```python
from build123d import *

# Parameters (mm, degrees)
SKETCH1_W           = 1.5875
SKETCH1_H           = 177.8
BOSS_EXTRUDE1_DEPTH = 304.8
CUT_EXTRUDE1_DEPTH  = 1.5875
FILLET1_R           = 6.35


with BuildPart() as part:
    # Sketch1 → Boss-Extrude1 (new body)
    with BuildSketch(Plane(origin=(0, 0, 0), x_dir=(1, 0, 0), z_dir=(0, 1, 0))):
        with Locations((0.79375, 88.9)):
            Rectangle(SKETCH1_W, SKETCH1_H)
    extrude(amount=BOSS_EXTRUDE1_DEPTH)

    # Sketch2 → Cut-Extrude1 (cut)
    with BuildSketch(Plane.ZY):
        Polygon((-177.8, 25.4), (0, 304.8), (-177.8, 304.8), align=None)
    extrude(amount=-CUT_EXTRUDE1_DEPTH, mode=Mode.SUBTRACT)

    # Fillet1
    fillet1_edges = [part.edges().sort_by_distance(p)[0] for p in [
        (0.79375, 25.4, -177.8),
        (0.79375, 304.8, 0),
        (0.79375, 0, -177.8),
        (0.79375, 0, 0),
    ]]
    fillet(fillet1_edges, radius=FILLET1_R)


solid = part.part
```
Geometry: final body of the model. Coordinates: model frame, mm. Coordinates: 2 decimals unless noted, no trailing zeros. Loops run counter-clockwise (first coordinate to the right, second up) from the corner with the lowest first, then second, coordinate; pieces in that order, holes last. Notation, with made-up numbers: (75, -19) -> (111, -19) arc R10 cw to (111, -5) -> close; hole circle Ø9 at (25.25, -17.75). An arc over 180 degrees is marked (long way). Use a Markdown table: item, result. Add a question column.
(1) Line query: line 1 along Y through (x, z) = (1.4, -74); line 2 along Y through (x, z) = (0.75, -12); line 3 along Z through (x, y) = (0.7, 122). Output: solid intervals per line, ascending.
(2) Section query A-A, the plane x = 1.3. Return loops of the section in (y, z), plus the area to 3 significant figures.
(3) Section query C-C, the plane y = 248.5. Return loops of the section in (x, z).
(4) Section query B-B, the plane z = -66.5. Return loops of the section in (x, y), plus the area to 3 significant figures.
Answer:
| question | item | result |
|---|---|---|
| 1 | line 1 | y = 0 to 188.51 |
| 1 | line 2 | y = 0 to 285.94 |
| 1 | line 3 | z = -116.33 to 0 |
| 2 | outline | (0, -171.45) arc R6.35 ccw to (6.35, -177.8) -> (23.55, -177.8) arc R6.35 ccw to (26.96, -176.81) -> (286.4, -11.71) arc R6.35 ccw to (282.99, 0) -> (6.35, 0) arc R6.35 ccw to (0, -6.35) -> close |
| 2 | area | 29,300 mm^2 |
| 3 | outline | (0, -35.83) -> (1.59, -35.83) -> (1.59, 0) -> (0, 0) -> close |
| 4 | outline | (0, 0) -> (1.59, 0) -> (1.59, 200.3) -> (0, 200.3) -> close |
| 4 | area | 318 mm^2 |
